```python
from build123d import *

# Parameters (mm, degrees)
F0_R     = 2.3876
F1_DEPTH = 5.08
F2_R     = 1.7526
F3_DEPTH = 8.89
F4_R     = 1.905
F5_DEPTH = 19.05
F6_SIZE  = 0.508
F7_W     = 8.721276
F7_H     = 1.003916
F8_DEPTH = 1.27


with BuildPart() as f1:
    # F0 (on Top) → F1 (new body)
    with BuildSketch(Plane.XY):
        Circle(F0_R)
    extrude(amount=F1_DEPTH)

    # F2 (on face) → F3 (join)
    with BuildSketch(Plane.XY.offset(5.08)):
        Circle(F2_R)
    extrude(amount=F3_DEPTH)

    # F4 (on face) → F5 (join)
    with BuildSketch(Plane(origin=(0, 0, 0), x_dir=(1, 0, 0), z_dir=(0, 0, -1))):
        Circle(F4_R)
    extrude(amount=F5_DEPTH)

    # F6
    f6_edges = [f1.edges().sort_by_distance(p)[0] for p in [
        (-1.905, 0, -19.05),
    ]]
    chamfer(f6_edges, length=F6_SIZE)

    # F7 (on face) → F8 (cut)
    with BuildSketch(Plane(origin=(0, 0, -19.05), x_dir=(1, 0, 0), z_dir=(0, 0, -1))):
        Rectangle(F7_W, F7_H)
    extrude(amount=-F8_DEPTH, mode=Mode.SUBTRACT)


solid = f1.part
```
Can you work these out from the model? Positions are in its coordinate system, mm. A direction names the side the tool comes from. Coordinates: 2 decimals unless noted, no trailing zeros. Loops run counter-clockwise (first coordinate to the right, second up) from the corner with the lowest first, then second, coordinate; pieces in that order, holes last. Notation, with made-up numbers: M 49,64 L 66,64 A10 ccw 66,79 Z; hole C 61.25,88.5 d7. An arc over 180 degrees is marked long. Put each result on its own line as item: value. Start each with the question number.
(1) Which directions (+Z, -Z, +X, -X, +Y, -Y) give clear straight access to the entire face, cutting with the end or side of a thin tool? Please do faces 1 (the face through (-0.41, 1.86, -9.14)), 2 (the face through (-0.028, 1.534, -18.912)), 3 (the face through (0, 0.502, -18)).
(2) I need wall thicknesses on probe 1 along X at (y, z) = (1.3, -7.5); probe 2 along Z at (x, y) = (1.8, 0.95); probe 3 along Z at (x, y) = (-0.3, 0.15). Which ranges of each line are inside material? Lowest first, please.
(3) Will these pins go through, and if not, where does the flat tip stop? pin 1 Ø1.4 at (x, z) = (0, -18.5) entering from -Y (3 decimals); pin 2 Ø1 at (x, z) = (-0.5, -18.5) entering from +Y (3 decimals); pin 3 Ø0.5 at (x, y) = (0.5, 0) entering from -Z.
(4) We'd pull the mould along Y, two halves only. Please class faces 4 (the face through (0, 0, -17.78)), 5 (the face through (-1, 2, 5.08)), 6 (the face through (0, -0.502, -18)), 7 (the face through (1.67, 0.53, 9.46)): +Y half, -Y half, draft (parallel to the pull), parting line (faces both ways), or undercut.
(5) Imagine slicing it at A-A on y = 0. List the corners of the cut face in (x, z) for me (3 decimals).
(6) Imagine slicing it at B-B on x = 0. List the corners of the cut face in (y, z) for me (3 decimals).
(7) Imagine slicing it at C-C on z = -10.5. List the corners of the cut face in (x, y) for me (3 decimals), and give its area (3 significant figures).
(8) Imagine slicing it at D-D on z = 7. List the corners of the cut face in (x, y) for me.
Worked answers:
1. face 1: -Z
1. face 2: -Z, +Y
1. face 3: -Z, +X, -X
2. probe 1: x = -1.39 to 1.39
2. probe 2: z = 0 to 5.08
2. probe 3: z = -17.78 to 13.97
3. pin 1: stops at y = -1.905
3. pin 2: stops at y = 1.905
3. pin 3: stops at z = -17.78
4. face 4: undercut
4. face 5: draft
4. face 6: undercut
4. face 7: parting line
5. outline: M -2.388,0 L -1.905,0 L -1.905,-17.78 L 1.905,-17.78 L 1.905,0 L 2.388,0 L 2.388,5.08 L 1.753,5.08 L 1.753,13.97 L -1.753,13.97 L -1.753,5.08 L -2.388,5.08 Z
6. outline: M -2.388,0 L -1.905,0 L -1.905,-18.542 L -1.397,-19.05 L -0.502,-19.05 L -0.502,-17.78 L 0.502,-17.78 L 0.502,-19.05 L 1.397,-19.05 L 1.905,-18.542 L 1.905,0 L 2.388,0 L 2.388,5.08 L 1.753,5.08 L 1.753,13.97 L -1.753,13.97 L -1.753,5.08 L -2.388,5.08 Z
7. outline: C 0,0 d3.81
7. area: 11.4 mm2
8. outline: C 0,0 d3.51
